Source: three-view drawing plus pictorial views. Frame: mm from the lowest corner of the part. A direction names the side the tool comes from. Give positions to 0.01 mm unless a question says otherwise; leave off trailing zeros. Order: outer loops, then holes, each group sorted by start corner. A loop starts at its lowest first (then second) coordinate and runs counter-clockwise, first axis right, second up. Notation, with made-up numbers: (29, 76) -> (53, 76) arc R34 cw to (53, 107) -> close; hole circle Ø2 at (21.5, 37). An arc over 180 degrees is marked (long way). Answer in a Markdown table with one row per item.
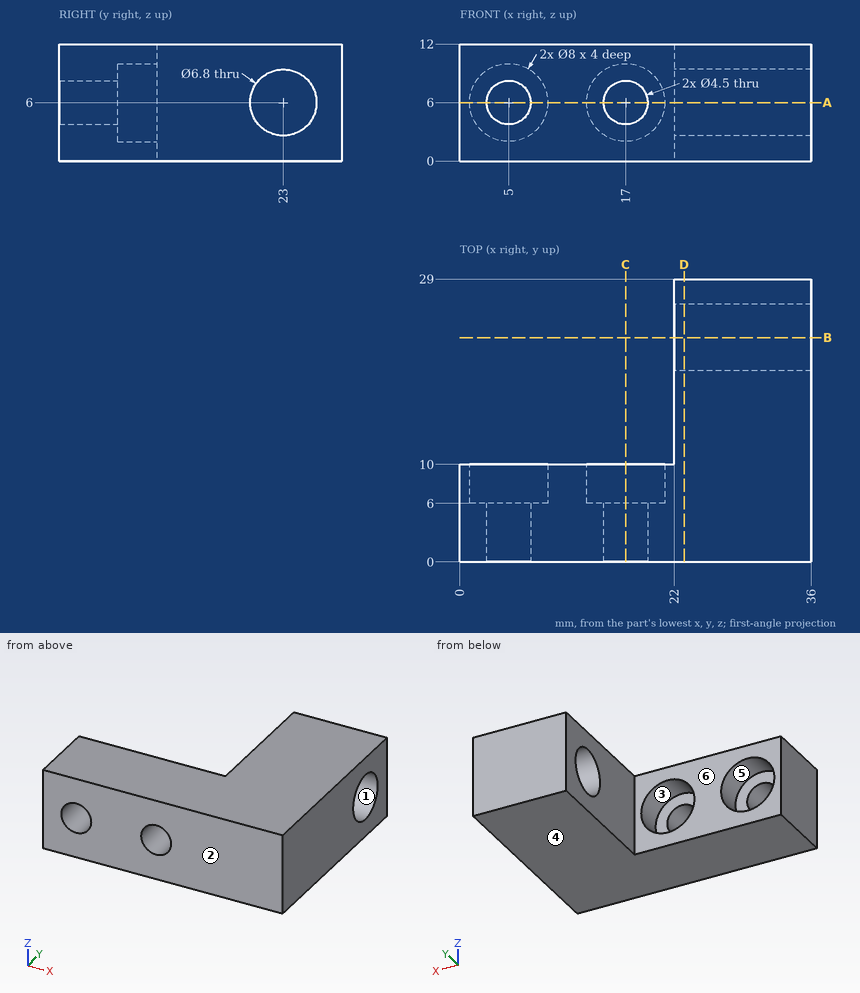
(1) Section query D-D (x = 23). Return the cut outline in (y, z), plus the area to 3 significant figures.
A:
| item | result |
|---|---|
| outline | (0, 0) -> (29, 0) -> (29, 12) -> (0, 12) -> close; hole circle Ø6.8 at (23, 6) |
| area | 312 mm^2 |
(2) First-contact query: pin 1 Ø8 at (x, y) = (20.5, 19) entering from -Z; pin 2 Ø2.5 at (x, z) = (3, 4.5) entering from +Y; pin 3 Ø2 at (y, z) = (20, 2.5) entering from -X. Flat tips, straight axial feed; report the tip coordinate or a pass-through.
A:
| item | result |
|---|---|
| pin 1 | stops at z = 0 |
| pin 2 | stops at y = 6 |
| pin 3 | stops at x = 22 |
(3) Access query for the marked faces 4, 5 and 6. Directions: +Z, -Z, +X, -X, +Y, -Y. A direction counts if a zero-diameter tool reaches every point of the face in a straight line with its end or side. Return the directions, or none.
A:
| item | result |
|---|---|
| face 4 | -Z, +X, -X, +Y, -Y |
| face 5 | +Y |
| face 6 | +Z, -Z, -X, +Y |
(4) Section query B-B (y = 23). Return the cut outline in (x, z).
A:
| item | result |
|---|---|
| outline | (22, 0) -> (36, 0) -> (36, 2.6) -> (22, 2.6) -> close; (22, 9.4) -> (36, 9.4) -> (36, 12) -> (22, 12) -> close |
(5) Section query A-A (z = 6). Return the cut outline in (x, y), plus the area to 3 significant figures.
A:
| item | result |
|---|---|
| outline | (0, 0) -> (2.75, 0) -> (2.75, 6) -> (1, 6) -> (1, 10) -> (0, 10) -> close; (7.25, 0) -> (14.75, 0) -> (14.75, 6) -> (13, 6) -> (13, 10) -> (9, 10) -> (9, 6) -> (7.25, 6) -> close; (19.25, 0) -> (36, 0) -> (36, 19.6) -> (22, 19.6) -> (22, 10) -> (21, 10) -> (21, 6) -> (19.25, 6) -> close; (22, 26.4) -> (36, 26.4) -> (36, 29) -> (22, 29) -> close |
| area | 413 mm^2 |
(6) Pull-direction query (Y, two-part tool) for the marked faces 1, 2 and 3; classes: +Y half, -Y half, draft (parallel to the pull), parting line (faces both ways), or undercut.
A:
| item | result |
|---|---|
| face 1 | undercut |
| face 2 | -Y half |
| face 3 | draft |
(7) Section query C-C (x = 17). Return the cut outline in (y, z), plus the area to 3 significant figures.
A:
| item | result |
|---|---|
| outline | (0, 0) -> (10, 0) -> (10, 2) -> (6, 2) -> (6, 3.75) -> (0, 3.75) -> close; (0, 8.25) -> (6, 8.25) -> (6, 10) -> (10, 10) -> (10, 12) -> (0, 12) -> close |
| area | 61.0 mm^2 |
(8) Ray query, probe 1 along X at (y, z) = (9.1, 6); probe 2 along X at (y, z) = (3.5, 6); probe 3 along Z at (x, y) = (5, 2). Return the intervals inside material, ascending.
A:
| item | result |
|---|---|
| probe 1 | x = 0 to 1, 9 to 13, 21 to 36 |
| probe 2 | x = 0 to 2.75, 7.25 to 14.75, 19.25 to 36 |
| probe 3 | z = 0 to 3.75, 8.25 to 12 |
